from build123d import *

# Parameters (mm, degrees)
SKETCH6_R           = 6.35
SKETCH6_R_2         = 53.34
BOSS_EXTRUDE1_DEPTH = 19.05
SKETCH10_R          = 50.8
SKETCH10_R_2        = 2.54
SKETCH10_R_3        = 1.524
CUT_EXTRUDE3_DEPTH  = 5.9436
CUT_EXTRUDE4_REACH  = 87.98
SKETCH11_R          = 12.7


with BuildPart() as part:
    # Sketch6 → Boss-Extrude1 (new body)
    with BuildSketch(Plane.XY):
        with Locations((-18.243354445, 50.123204393)):
            Circle(SKETCH6_R)
        Circle(SKETCH6_R_2)
        with Locations((-34.286291101, 40.860810596)):
            Circle(SKETCH6_R)
        with Locations((-46.193795038, 26.67)):
            Circle(SKETCH6_R)
        with Locations((-52.529645546, 9.262393797)):
            Circle(SKETCH6_R)
        with Locations((-52.529645546, -9.262393797)):
            Circle(SKETCH6_R)
        with Locations((-46.193795038, -26.67)):
            Circle(SKETCH6_R)
        with Locations((-34.286291101, -40.860810596)):
            Circle(SKETCH6_R)
        with Locations((-18.243354445, -50.123204393)):
            Circle(SKETCH6_R)
        with Locations((0, -53.34)):
            Circle(SKETCH6_R)
        with Locations((18.243354445, -50.123204393)):
            Circle(SKETCH6_R)
        with Locations((34.286291101, -40.860810596)):
            Circle(SKETCH6_R)
        with Locations((46.193795038, -26.67)):
            Circle(SKETCH6_R)
        with Locations((52.529645546, -9.262393797)):
            Circle(SKETCH6_R)
        with Locations((52.529645546, 9.262393797)):
            Circle(SKETCH6_R)
        with Locations((46.193795038, 26.67)):
            Circle(SKETCH6_R)
        with Locations((34.286291101, 40.860810596)):
            Circle(SKETCH6_R)
        with Locations((18.243354445, 50.123204393)):
            Circle(SKETCH6_R)
        with Locations((0, 53.34)):
            Circle(SKETCH6_R)
    extrude(amount=BOSS_EXTRUDE1_DEPTH)

    # Sketch10 → Cut-Extrude3 (cut, symmetric)
    with BuildSketch(Plane.XY.offset(9.525)):
        Circle(SKETCH10_R)
        with Locations((0, 44.45)):
            Circle(SKETCH10_R_2, mode=Mode.SUBTRACT)
        with Locations((38.494829198, 22.225)):
            Circle(SKETCH10_R_2, mode=Mode.SUBTRACT)
        with Locations((38.494829198, -22.225)):
            Circle(SKETCH10_R_2, mode=Mode.SUBTRACT)
        with Locations((0, -44.45)):
            Circle(SKETCH10_R_2, mode=Mode.SUBTRACT)
        with Locations((-38.494829198, -22.225)):
            Circle(SKETCH10_R_2, mode=Mode.SUBTRACT)
        with Locations((-38.494829198, 22.225)):
            Circle(SKETCH10_R_2, mode=Mode.SUBTRACT)
        with Locations((0, 15.24)):
            Circle(SKETCH10_R_3, mode=Mode.SUBTRACT)
        with Locations((13.198227154, -7.62)):
            Circle(SKETCH10_R_3, mode=Mode.SUBTRACT)
        with Locations((-13.198227154, -7.62)):
            Circle(SKETCH10_R_3, mode=Mode.SUBTRACT)
    extrude(amount=CUT_EXTRUDE3_DEPTH, both=True, mode=Mode.SUBTRACT)

    # Sketch11 → Cut-Extrude4 (cut, up to next)
    with BuildSketch(Plane.XY.offset(19.05), mode=Mode.PRIVATE) as cut_extrude4_sk1:
        Circle(SKETCH11_R)
    cut_extrude4_tool1 = extrude(cut_extrude4_sk1.sketch, amount=-CUT_EXTRUDE4_REACH, mode=Mode.PRIVATE) & part.part
    add(cut_extrude4_tool1.solids().sort_by_distance((0, 0, 19.05))[0], mode=Mode.SUBTRACT)


solid = part.part
Geometry check sheet. Reference: the model listing, model coordinates, mm. A direction names the side the tool comes from. Give positions to 0.01 mm unless a question says otherwise; leave off trailing zeros. Order: outer loops, then holes, each group sorted by start corner. A loop starts at its lowest first (then second) coordinate and runs counter-clockwise, first axis right, second up. Notation, with made-up numbers: (73.5, 61.25) - (126.5, 61.25) arc R15 ccw to (126.5, 77.25) - close; hole circle Ø6 at (58, 82.25). An arc over 180 degrees is marked (long way). Use one line per item in the form item = value.
1) Sectioned sample at B-B (y = -7.62). Record the boundary of the cut face in (x, z), and give its area (3 significant figures).
Working result:
outline = (-58.66, 0) - (58.66, 0) - (58.66, 19.05) - (10.16, 19.05) - (10.16, 15.47) - (11.67, 15.47) - (11.67, 3.58) - (-11.67, 3.58) - (-11.67, 15.47) - (-10.16, 15.47) - (-10.16, 19.05) - (-58.66, 19.05) - close; hole (-50.23, 3.58) - (-14.72, 3.58) - (-14.72, 15.47) - (-50.23, 15.47) - close; hole (14.72, 3.58) - (50.23, 3.58) - (50.23, 15.47) - (14.72, 15.47) - close
area = 1,040 mm^2
2) Material ranges on probe 1 along Y at (x, z) = (0, 9.25); probe 2 along Z at (x, y) = (29, 5.5); probe 3 along Y at (x, z) = (-37.5, 3.75), recorded low to high. Write a range as from..to.
Working result:
probe_1 = -59.69..-50.8, -46.99..-41.91, 13.72..16.76, 41.91..46.99, 50.8..59.69
probe_2 = 0..3.58, 15.47..19.05
probe_3 = -46.34..-34.27, -24.56..-19.89, 19.89..24.56, 34.27..46.34
3) Sectioned sample at D-D (y = 26.67). Record the boundary of the cut face in (x, z).
Working result:
outline = (-52.54, 0) - (52.54, 0) - (52.54, 19.05) - (-52.54, 19.05) - close; hole (-43.24, 3.58) - (43.24, 3.58) - (43.24, 15.47) - (-43.24, 15.47) - close
4) Depth check by flat-ended pin: pin 1 Ø1.5 at (y, z) = (-28.5, 10) entering from -X; pin 2 Ø4 at (x, z) = (33.5, 9) entering from -Y. Enter the tip coordinate at first touch or a pass-through.
Working result:
pin_1 = -52.45
pin_2 = -47.21
5) Sectioned sample at C-C (z = 5). Count the separate pieces of the cut face and the enclosed holes in it, and give its area (3 significant figures).
Working result:
separate_pieces = 10
enclosed_holes = 1
area = 2,140 mm^2
6) Access from +Z, -Z, +X, -X, +Y, -Y to the whole of each face (thin tool, end or side, straight path). Record for faces 1 (the face through (9.303, 52.522, 9.392)), 2 (the face through (-0.33, 46.97, 9.44)), 3 (the face through (40.89, 34.25, 9.39)).
Working result:
face_1 = +Z, -Z, +Y
face_2 = none
face_3 = +Z, -Z
7) Sectioned sample at A-A (x = 0). Record the boundary of the cut face in (y, z).
Working result:
outline = (-59.69, 0) - (59.69, 0) - (59.69, 19.05) - (12.7, 19.05) - (12.7, 15.47) - (13.72, 15.47) - (13.72, 3.58) - (-41.91, 3.58) - (-41.91, 15.47) - (-12.7, 15.47) - (-12.7, 19.05) - (-59.69, 19.05) - close; hole (-50.8, 3.58) - (-46.99, 3.58) - (-46.99, 15.47) - (-50.8, 15.47) - close; hole (16.76, 3.58) - (41.91, 3.58) - (41.91, 15.47) - (16.76, 15.47) - close; hole (46.99, 3.58) - (50.8, 3.58) - (50.8, 15.47) - (46.99, 15.47) - close
8) Draft check along X on faces 4 (the face through (-1, 1, 0)), 5 (the face through (9.222, -52.537, 9.392)), 6 (the face through (53.34, -0.04, 9.39)). Enter one of: released by +X, released by -X, zero draft, split by the parting line, or undercut.
Working result:
face_4 = zero draft
face_5 = undercut
face_6 = released by +X
